```python
from build123d import *

# Parameters (mm, degrees)
F0_R     = 52.25
F0_R_2   = 1.225
F0_R_3   = 45
F1_DEPTH = 6
F2_R     = 1.5
F3_DEPTH = 5.9
F4_R     = 0.5


with BuildPart() as f1:
    # F0 (on Top) → F1 (new body)
    with BuildSketch(Plane.XY):
        Circle(F0_R)
        with Locations((-46.601769, -15.141833)):
            Circle(F0_R_2, mode=Mode.SUBTRACT)
        with Locations((0, -49)):
            Circle(F0_R_2, mode=Mode.SUBTRACT)
        with Locations((46.601769, -15.141833)):
            Circle(F0_R_2, mode=Mode.SUBTRACT)
        with Locations((-28.801477, 39.641833)):
            Circle(F0_R_2, mode=Mode.SUBTRACT)
        Circle(F0_R_3, mode=Mode.SUBTRACT)
        with Locations((28.801477, 39.641833)):
            Circle(F0_R_2, mode=Mode.SUBTRACT)
    extrude(amount=F1_DEPTH)

    # F2
    f2_edges = [f1.edges().sort_by_distance(p)[0] for p in [
        (-45, 0, 6),
    ]]
    fillet(f2_edges, radius=F2_R)

    # F0 (on Top) → F3 (join)
    with BuildSketch(Plane.XY):
        Circle(F0_R)
        with Locations((-46.601769, -15.141833)):
            Circle(F0_R_2, mode=Mode.SUBTRACT)
        with Locations((0, -49)):
            Circle(F0_R_2, mode=Mode.SUBTRACT)
        with Locations((46.601769, -15.141833)):
            Circle(F0_R_2, mode=Mode.SUBTRACT)
        with Locations((-28.801477, 39.641833)):
            Circle(F0_R_2, mode=Mode.SUBTRACT)
        Circle(F0_R_3, mode=Mode.SUBTRACT)
        with Locations((28.801477, 39.641833)):
            Circle(F0_R_2, mode=Mode.SUBTRACT)
    extrude(amount=F3_DEPTH)

    # F4
    f4_edges = [f1.edges().sort_by_distance(p)[0] for p in [
        (-45, 0, 0),
        (-52.25, 0, 0),
        (-52.25, 0, 6),
    ]]
    fillet(f4_edges, radius=F4_R)


solid = f1.part
```
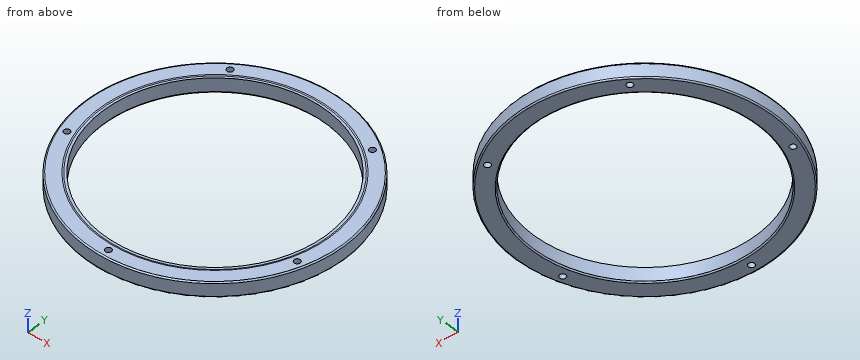
Design review of the part built by this model. Coordinates are the model's own, in mm. Give positions to 0.01 mm unless a question says otherwise; leave off trailing zeros. Write each loop counter-clockwise with the first axis right and the second up, starting at its lowest first coordinate (ties: lowest second). Pieces come first, ordered by that corner, then holes. Notation, with made-up numbers: (-38, -17) -> (-15, -17) arc R22 cw to (-15, -5) -> close; hole circle Ø8 at (-18.5, -31.75). An arc over 180 degrees is marked (long way). Answer in a Markdown table with one row per item.
(1) Clearance check with a flat-ended pin moving along its axis: pin 1 (2 mm diameter, centred on x = -4.5, z = 1.5, fed in from +Y). State where the tip first meets the part, or that it passes through.
Results:
| item | result |
|---|---|
| pin 1 | y = 52.13 |
(2) To check wall thickness, follow probe 1 along Y at (x, z) = (0, 2.8) (3 decimals); probe 2 along Y at (x, z) = (0.5, 1.4); probe 3 along Y at (x, z) = (-15, 5). State the ranges of each line that lie inside material, in increasing order.
Results:
| item | result |
|---|---|
| probe 1 | -52.25 to -50.225, -47.775 to -45, 45 to 52.25 |
| probe 2 | -52.25 to -50.12, -47.88 to -45, 45 to 52.25 |
| probe 3 | -50.05 to -42.43, 42.43 to 50.05 |
(3) Consider section C-C (z = 3). State the section outline as (x, y) points (3 decimals).
Results:
| item | result |
|---|---|
| outline | circle Ø104.5 at (0, 0); hole circle Ø2.45 at (-46.602, -15.142); hole circle Ø90 at (0, 0); hole circle Ø2.45 at (-28.801, 39.642); hole circle Ø2.45 at (0, -49); hole circle Ø2.45 at (28.801, 39.642); hole circle Ø2.45 at (46.602, -15.142) |
(4) Consider section A-A (x = 0). State the section outline as (y, z) points (3 decimals), then the cut area to 3 significant figures.
Results:
| item | result |
|---|---|
| outline | (-52.25, 0.5) arc R0.5 ccw to (-51.75, 0) -> (-50.225, 0) -> (-50.225, 6) -> (-51.75, 6) arc R0.5 ccw to (-52.25, 5.5) -> close; (-47.775, 0) -> (-45.5, 0) arc R0.5 ccw to (-45, 0.5) -> (-45, 5.9) -> (-45.961, 5.9) arc R1.5 ccw to (-46.5, 6) -> (-47.775, 6) -> close; (45, 0.5) arc R0.5 ccw to (45.5, 0) -> (51.75, 0) arc R0.5 ccw to (52.25, 0.5) -> (52.25, 5.5) arc R0.5 ccw to (51.75, 6) -> (46.5, 6) arc R1.5 ccw to (45.961, 5.9) -> (45, 5.9) -> close |
| area | 71.8 mm2 |
(5) Consider section B-B (y = 0). State the section outline as (x, z) points.
Results:
| item | result |
|---|---|
| outline | (-52.25, 0.5) arc R0.5 ccw to (-51.75, 0) -> (-45.5, 0) arc R0.5 ccw to (-45, 0.5) -> (-45, 5.9) -> (-45.96, 5.9) arc R1.5 ccw to (-46.5, 6) -> (-51.75, 6) arc R0.5 ccw to (-52.25, 5.5) -> close; (45, 0.5) arc R0.5 ccw to (45.5, 0) -> (51.75, 0) arc R0.5 ccw to (52.25, 0.5) -> (52.25, 5.5) arc R0.5 ccw to (51.75, 6) -> (46.5, 6) arc R1.5 ccw to (45.96, 5.9) -> (45, 5.9) -> close |
